Check sheet for the modelled part. Datum: model origin and axes. Units: mm. Face numbers are marked on the shaded views. A direction names the side the tool comes from. Round coordinates to 2 decimals unless told otherwise and drop trailing zeros. Loops run counter-clockwise (first coordinate to the right, second up) from the corner with the lowest first, then second, coordinate; pieces in that order, holes last. Notation, with made-up numbers: (-15, 23.5) - (25, 23.5) arc R21 ccw to (25, 62.5) - close; hole circle Ø7 at (74.25, 60). An arc over 180 degrees is marked (long way). Return JSON: item names as keys, results as strings.
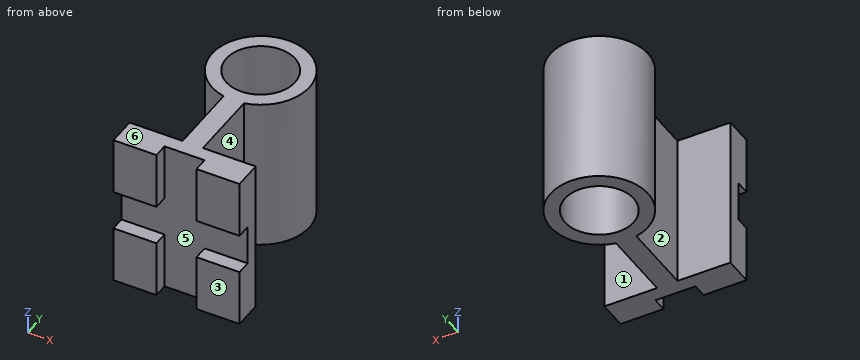
from build123d import *

# Parameters (mm, degrees)
SKETCH1_R           = 12
BOSS_EXTRUDE1_DEPTH = 54
SKETCH2_W           = 14
SKETCH2_H           = 5
CUT_EXTRUDE1_DEPTH  = 44


with BuildPart() as part:
    # Sketch1 → Boss-Extrude1 (new body)
    with BuildSketch(Plane.XY):
        with BuildLine():
            Line((-22, 0), (-7, 0))
            Line((-7, 0), (-7, 5))
            Line((-7, 5), (7, 5))
            Line((7, 5), (7, 0))
            Line((7, 0), (22, 0))
            Line((22, 0), (22, 10))
            Line((22, 10), (3.575995422, 10))
            Line((3.575995422, 10), (3.575995422, 35.405163338))
            ThreePointArc((3.575995422, 35.405163338), (0.016529647, 69.028346048), (-3.542936129, 35.405163338))
            Line((-3.542936129, 35.405163338), (-3.542936129, 10.023734162))
            Line((-3.542936129, 10.023734162), (-22, 10))
            Line((-22, 10), (-22, 0))
        make_face()
        with Locations((0.016529647, 52.028346048)):
            Circle(SKETCH1_R, mode=Mode.SUBTRACT)
    extrude(amount=-BOSS_EXTRUDE1_DEPTH)

    # Sketch2 → Cut-Extrude1 (cut)
    with BuildSketch(Plane(origin=(22, 0, 0), x_dir=(0, 0, -1), z_dir=(1, 0, 0))):
        with Locations((27, 2.5)):
            Rectangle(SKETCH2_W, SKETCH2_H)
    extrude(amount=-CUT_EXTRUDE1_DEPTH, mode=Mode.SUBTRACT)


solid = part.part
Q1. Sectioned sample at D-D (x = -6). Enter the section's corners in (y, z), plus the area to 3 significant figures.
Answer key:
{"outline": "(5, -54) - (10.02, -54) - (10.02, 0) - (5, 0) - close; (36.13, -54) - (41.65, -54) - (41.65, 0) - (36.13, 0) - close; (62.41, -54) - (67.93, -54) - (67.93, 0) - (62.41, 0) - close", "area": "867 mm²"}
Q2. Draft check along X on the marked faces 4, 5 and 6. Enter one of: released by +X, released by -X, zero draft, split by the parting line, or undercut.
Answer key:
{"face 4": "released by +X", "face 5": "undercut", "face 6": "zero draft"}
Q3. Scan lines: probe 1 along Y at (x, z) = (-0.5, -30.5); probe 2 along Y at (x, z) = (-7.5, -13); probe 3 along Y at (x, z) = (9, -6). Record each from-to range of solid material in increasing order. Write a range as [from, to].
Answer key:
{"probe 1": "y = [5, 40.04], [64.02, 69.02]", "probe 2": "y = [0, 10.02], [36.78, 42.67], [61.38, 67.28]", "probe 3": "y = [0, 10], [37.6, 44.07], [59.98, 66.46]"}
Q4. Tool access check on the marked faces 1, 2 and 3. Record the directions out of +Z, -Z, +X, -X, +Y, -Y that give a thin tool (end or side, any length) a straight path to the whole face; none if there is none.
Answer key:
{"face 1": "+Z, -Z, +X", "face 2": "+Z, -Z, -X", "face 3": "+Z, -Z, +X, -X, -Y"}
Q5. Sectioned sample at A-A (x = 15.5). Enter the section's corners in (y, z).
Answer key:
{"outline": "(0, -54) - (10, -54) - (10, 0) - (0, 0) - (0, -20) - (5, -20) - (5, -34) - (0, -34) - close; (45.01, -54) - (59.05, -54) - (59.05, 0) - (45.01, 0) - close"}
Q6. Sectioned sample at C-C (y = 60). Enter the section's corners in (x, z).
Answer key:
{"outline": "(-15, -54) - (-8.95, -54) - (-8.95, 0) - (-15, 0) - close; (8.99, -54) - (15.03, -54) - (15.03, 0) - (8.99, 0) - close"}
Q7. Depth check by flat-ended pin: P1, Ø1, axis at x = 13.5, z = -32, coming from the +Y side; P2, Ø1, axis at x = 13, z = -25, coming from the -Y side; P3, Ø20.5, axis at x = 17, z = -35, coming from the +Y side. Enter the tip coordinate at first touch or a pass-through.
Answer key:
{"P1": "stops at y = 63", "P2": "stops at y = 5", "P3": "stops at y = 67.64"}
Q8. Sectioned sample at B-B (z = -23.5). Enter the section's corners in (x, y), plus the area to 3 significant figures.
Answer key:
{"outline": "(-22, 5) - (22, 5) - (22, 10) - (3.58, 10) - (3.58, 35.41) arc R17 ccw (long way) to (-3.54, 35.41) - (-3.54, 10.02) - (-22, 10) - close; hole circle Ø24 at (0.02, 52.03)", "area": "855 mm²"}
